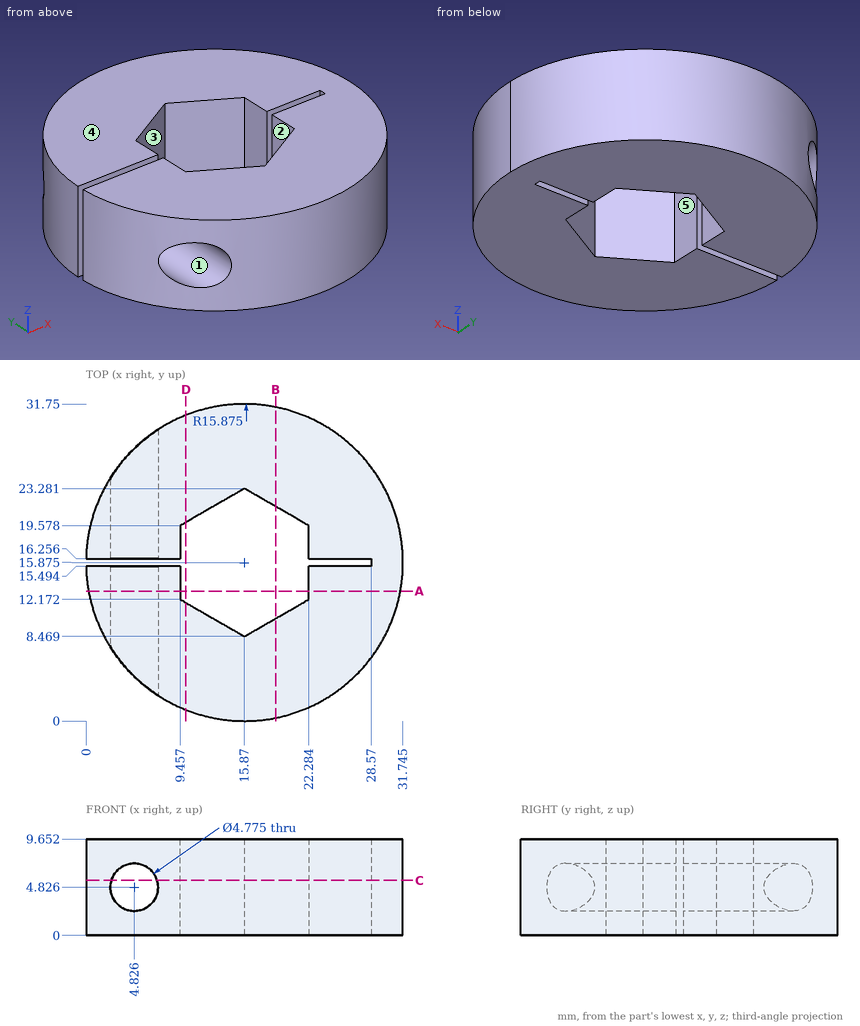
Verification items for this drawing (mm, ordinates from the low corner). A direction names the side the tool comes from. Give positions to 0.01 mm unless a question says otherwise; leave off trailing zeros. Loops run counter-clockwise (first coordinate to the right, second up) from the corner with the lowest first, then second, coordinate; pieces in that order, holes last. Notation, with made-up numbers: M 40,84 L 94,84 A8 cw 94,95 Z; hole C 86,16.25 d2. An arc over 180 degrees is marked long. Answer as a JSON object with one key per item and string values. Group by question number.
Item 1: Sectioned sample at D-D on x = 10. Record the boundary of the cut face in (y, z) (1 decimal), plus the area to 3 significant figures.
Item 2: Gauge pin test, flat ends, axial feed: pin 1 (3 mm diameter, centred on x = 28, z = 3.5, fed in from +Y) (1 decimal); pin 2 (2 mm diameter, centred on y = 9.5, z = 2.5, fed in from -X); pin 3 (3 mm diameter, centred on x = 4.826, z = 4.826, fed in from -Y); pin 4 (1.7 mm diameter, centred on y = 17.5, z = 5.5, fed in from +X). Record the tip position at first contact, or that the pin passes through.
Item 3: Sectioned sample at B-B on x = 19. Record the boundary of the cut face in (y, z).
Item 4: Access from +Z, -Z, +X, -X, +Y, -Y to the whole of each face (thin tool, end or side, straight path). Record for the marked faces 1 and 2.
Item 5: Sectioned sample at C-C on z = 5.5. Give the number of separate pieces and of enclosed holes in the cut face, plus the area to 3 significant figures.
Item 6: Material ranges on L1, parallel to X at y = 15, z = 6 (1 decimal); L2, parallel to X at y = 13, z = 4.5 (1 decimal); L3, parallel to Y at x = 14, z = 6, recorded low to high.
Item 7: Mould release check, pull along X, two halves, no side actions. Record for the marked faces 3, 4 and 5: pulls with the +X half, pulls with the -X half, needs draft (parallel to the pull), parting line crosses it, or undercut.
Item 8: Sectioned sample at A-A on y = 13. Record the boundary of the cut face in (x, z) (1 decimal), plus the area to 3 significant figures.
Findings below:
{
 "1": {"outline": "M 1.1,0 L 11.9,0 L 11.9,9.7 L 1.1,9.7 Z; M 19.9,0 L 30.6,0 L 30.6,9.7 L 19.9,9.7 Z", "area": "207 mm2"},
 "2": {"pin 1": "y = 27.7", "pin 2": "x = 0.93", "pin 3": "through", "pin 4": "x = 31.73"},
 "3": {"outline": "M 0.31,0 L 10.28,0 L 10.28,9.65 L 0.31,9.65 Z; M 21.47,0 L 31.44,0 L 31.44,9.65 L 21.47,9.65 Z"},
 "4": {"face 1": "+Y, -Y", "face 2": "+Z, -Z"},
 "5": {"separate pieces": "3", "enclosed holes": "0", "area": "538 mm2"},
 "6": {"L1": "0 to 2.7, 6.9 to 9.5, 22.3 to 31.7", "L2": "0.3 to 2.5, 7.2 to 9.5, 22.3 to 31.5", "L3": "0.11 to 9.55, 22.2 to 31.64"},
 "7": {"face 3": "undercut", "face 4": "needs draft", "face 5": "undercut"},
 "8": {"outline": "M 0.3,0 L 9.5,0 L 9.5,9.7 L 0.3,9.7 Z; M 22.3,0 L 31.5,0 L 31.5,9.7 L 22.3,9.7 Z; hole C 4.8,4.8 d4.8", "area": "160 mm2"}
}
